The listing builds one solid part. Answer for the finished solid, in the listing's coordinates (mm). A direction names the side the tool comes from. Coordinates: 2 decimals unless noted, no trailing zeros. Loops run counter-clockwise (first coordinate to the right, second up) from the corner with the lowest first, then second, coordinate; pieces in that order, holes last. Notation, with made-up numbers: (-25.75, 42.5) - (2.25, 42.5) arc R34 cw to (2.25, 76.5) - close; hole circle Ø5 at (-28, 49.5). An arc over 180 degrees is marked (long way). Write each question's results on one line, items separated by ' | '. Start each with the question number.
(1) Find section D-D on x = -40.5. Determine the outline of the cut face in (y, z).
(2) Find section C-C on z = 15.5. Determine the outline of the cut face in (x, y).
(3) Determine the mould class of faces 6 (the flat face through (50, 38.7, 10.5)), 7 (the cylindrical face through (-26.2, 5.1, -6.6)), 8 (the flat face through (-1, 5, -20)) for opening direction Z: released by +Z, released by -Z, zero draft, split by the parting line, or undercut.
(4) For faces 1 (the flat face through (5.2, 66, -5)), 2 (the flat face through (-7, 59, 1)), 3 (the flat face through (-5, 64, 11)), 4 (the flat face through (7, 59, -1)), 5 (the flat face through (-1, 60, -11)), determine the directions among +Z, -Z, +X, -X, +Y, -Y from which every point of the face is accessible in a straight line to the end or side of a thin tool.
(5) Consider line 1 (X direction, y = 2, z = -5); line 2 (X direction, y = 56.5, z = 3); line 3 (Y direction, x = 0, z = -1). Determine where each line is inside the solid, lowest interval first. Write a range as from..to.
(6) Find section A-A on z = -8.5. Determine the outline of the cut face in (x, y).
(7) Given pin 1 Ø1.5 at (x, y) = (28.5, 45) entering from -Z; pin 2 Ø11 at (y, z) = (61.5, -5.5) entering from +X; pin 3 Ø4 at (x, z) = (1, -3.5) entering from +Y; pin 4 Ø3.5 at (x, z) = (25, -5) entering from -Y, each flat-ended and moving along its own axis, determine where each tip first touches the part or whether it passes through.
(8) Find section B-B on x = 25. Determine the outline of the cut face in (y, z).
from build123d import *

# Parameters (mm, degrees)
SKETCH3_W           = 100
SKETCH3_H           = 40
BOSS_EXTRUDE1_DEPTH = 10
SKETCH4_W           = 100
SKETCH4_H           = 10
BOSS_EXTRUDE2_DEPTH = 90
SKETCH5_R           = 2
CUT_EXTRUDE1_DEPTH  = 90
SKETCH7_W           = 10
SKETCH7_H           = 12
CUT_EXTRUDE3_DEPTH  = 10
BOSS_EXTRUDE3_DEPTH = 23
SKETCH9_W           = 10
SKETCH9_H           = 2
BOSS_EXTRUDE5_DEPTH = 12
SKETCH12_W          = 2
SKETCH12_H          = 7
CUT_EXTRUDE6_DEPTH  = 12
SKETCH13_W          = 10
SKETCH13_H          = 12
CUT_EXTRUDE7_DEPTH  = 10


with BuildPart() as part:
    # Sketch3 → Boss-Extrude1 (new body)
    with BuildSketch(Plane(origin=(0, 0, 0), x_dir=(1, 0, 0), z_dir=(0, 1, 0))):
        Rectangle(SKETCH3_W, SKETCH3_H)
    extrude(amount=BOSS_EXTRUDE1_DEPTH)

    # Sketch4 → Boss-Extrude2 (add)
    with BuildSketch(Plane(origin=(0, 10, 0), x_dir=(1, 0, 0), z_dir=(0, 1, 0))):
        with Locations((0, -15)):
            Rectangle(SKETCH4_W, SKETCH4_H)
    extrude(amount=BOSS_EXTRUDE2_DEPTH)

    # Sketch5 → Cut-Extrude1 (cut)
    with BuildSketch(Plane(origin=(0, 10, 0), x_dir=(1, 0, 0), z_dir=(0, 1, 0))):
        with Locations(Location((-25, 5, 0), (0, 0, 270))):
            Circle(SKETCH5_R)
        with Locations(Location((25, 5, 0), (0, 0, 270))):
            Circle(SKETCH5_R)
    extrude(amount=-CUT_EXTRUDE1_DEPTH, mode=Mode.SUBTRACT)

    # Sketch7 → Cut-Extrude3 (cut)
    with BuildSketch(Plane(origin=(0, 0, 10), x_dir=(-1, 0, 0), z_dir=(0, 0, -1))):
        with Locations((0, 60)):
            Rectangle(SKETCH7_W, SKETCH7_H)
    extrude(amount=-CUT_EXTRUDE3_DEPTH, mode=Mode.SUBTRACT)

    # Sketch8 → Boss-Extrude3 (add)
    with BuildSketch(Plane(origin=(0, 0, 10), x_dir=(-1, 0, 0), z_dir=(0, 0, -1))):
        Polygon((-5, 54), (-5, 66), (-7, 66), (-7, 52), (7, 52), (7, 66), (5, 66), (5, 54), align=None)
    extrude(amount=BOSS_EXTRUDE3_DEPTH)

    # Sketch9 → Boss-Extrude5 (add)
    with BuildSketch(Plane(origin=(0, 54, 0), x_dir=(1, 0, 0), z_dir=(0, 1, 0))):
        with Locations((0, 12)):
            Rectangle(SKETCH9_W, SKETCH9_H)
    extrude(amount=BOSS_EXTRUDE5_DEPTH)

    # Sketch12 → Cut-Extrude6 (cut)
    with BuildSketch(Plane(origin=(0, 66, 0), x_dir=(1, 0, 0), z_dir=(0, 1, 0))):
        with Locations((-6, 7.5)):
            Rectangle(SKETCH12_W, SKETCH12_H)
    extrude(amount=-CUT_EXTRUDE6_DEPTH, mode=Mode.SUBTRACT)

    # Sketch13 → Cut-Extrude7 (cut)
    with BuildSketch(Plane(origin=(0, 0, 10), x_dir=(-1, 0, 0), z_dir=(0, 0, -1))):
        with Locations((0, 72)):
            Rectangle(SKETCH13_W, SKETCH13_H)
    extrude(amount=-CUT_EXTRUDE7_DEPTH, mode=Mode.SUBTRACT)


solid = part.part
Values:
1) outline: (0, -20) - (10, -20) - (10, 10) - (100, 10) - (100, 20) - (0, 20) - close
2) outline: (-50, 0) - (50, 0) - (50, 100) - (-50, 100) - close; hole (-5, 54) - (5, 54) - (5, 78) - (-5, 78) - close
3) face 6: zero draft | face 7: undercut | face 8: released by -Z
4) face 1: -Z, +X, -X, +Y | face 2: -Z, -X, +Y | face 3: +Z | face 4: -Z, +X, +Y | face 5: -X, +Y
5) line 1: x = -50..-27, -23..23, 27..50 | line 2: x = -7..-5, 5..7 | line 3: y = 0..10, 52..54
6) outline: (-50, 0) - (50, 0) - (50, 10) - (-50, 10) - close; (-7, 52) - (7, 52) - (7, 66) - (5, 66) - (5, 54) - (-7, 54) - close
7) pin 1: stops at z = 10 | pin 2: stops at x = 7 | pin 3: stops at y = 54 | pin 4: passes through
8) outline: (0, -20) - (10, -20) - (10, -7) - (0, -7) - close; (0, -3) - (10, -3) - (10, 10) - (100, 10) - (100, 20) - (0, 20) - close
